Autodesk Inventor part; units mm, degrees
ref_plane "YZ Plane" through (0, 0, 0) normal (1, 0, 0) x (0, 1, 0)
ref_plane "XZ Plane" through (0, 0, 0) normal (0, 1, 0) x (-1, 0, 0)
ref_plane "XY Plane" through (0, 0, 0) normal (0, 0, 1) x (1, 0, 0)
sketch "Sketch1" plane through (0, 0, 0) normal (0, 0, 1) x (1, 0, 0)
  circle A0 centre (0, 0) radius 19
  dimension "d0" = 38
extrude "Extrusion1" add sketch "Sketch1" along normal blind 59.1
sketch "Sketch2" plane through (0, 0, 59.1) normal (0, 0, 1) x (1, 0, 0)
  circle A0 centre (0, 0) radius 16
  dimension "d3" = 32
extrude "Extrusion2" add sketch "Sketch2" along normal blind 41.9
sketch "Sketch3" plane through (0, 0, 101) normal (0, 0, 1) x (1, 0, 0)
  circle A0 centre (0, 0) radius 10
  dimension "d6" = 20
extrude "Extrusion3" add sketch "Sketch3" along normal blind 3
sketch "Sketch4" plane through (0, 0, 104) normal (0, 0, 1) x (1, 0, 0)
  circle A0 centre (0, 0) radius 3
  dimension "d9" = 6
extrude "Extrusion4" add sketch "Sketch4" along normal blind 15.5
sketch "Sketch5" plane through (0, 0, 104) normal (0, 0, 1) x (1, 0, 0)
  line L0 (-9, -9) -> (9, -9) construction
  line L1 (9, -9) -> (9, 9) construction
  line L2 (9, 9) -> (-9, 9) construction
  line L3 (-9, 9) -> (-9, -9) construction
  line L4 (-9, -9) -> (9, 9) construction
  line L5 (9, -9) -> (-9, 9) construction
  circle A0 centre (9, 9) radius 1.5
  circle A1 centre (9, -9) radius 1.5
  circle A2 centre (-9, -9) radius 1.5
  circle A3 centre (-9, 9) radius 1.5
  point P0 (0, 0)
  dimension "d12" = 18
  dimension "d13" = 18
  dimension "d14" = 3
  dimension "d15" = 3
  dimension "d16" = 3
  dimension "d17" = 3
extrude "Extrusion5" cut sketch "Sketch5" against normal blind 25
sketch "Sketch6" plane through (0, 0, 101) normal (0, 0, 1) x (1, 0, 0)
  circle A0 centre (0, 0) radius 3
  circle A1 centre (0, 0) radius 10
  line L0 (-4.3589, -9) -> (4.3589, -9)
  line L1 (-4.3589, 9) -> (4.3589, 9)
  dimension "d20" = 18
extrude "Extrusion6" cut sketch "Sketch6" along normal through all contours L1 A1 | A1 L0
properties part number "12RPM Gear Motor"
Read the model definition and answer for the solid it produces. Units are mm, in the model's axes. A direction names the side the tool comes from. Give positions to 0.01 mm unless a question says otherwise; leave off trailing zeros. Write each loop counter-clockwise with the first axis right and the second up, starting at its lowest first coordinate (ties: lowest second). Pieces come first, ordered by that corner, then holes. Notation, with made-up numbers: (-28.5, -20) - (-0.5, -20) arc R27 ccw to (-0.5, 17) - close; hole circle Ø11 at (-11.5, 89.5). An arc over 180 degrees is marked (long way). Use CSV: the item, a comma, the result in double quotes. Start each with the question number.
(1) Find section C-C (z = 98). Give the vertices of the cut face in (x, y), plus the area to 3 significant figures.
(2) Find section B-B (x = 0). Give the vertices of the cut face in (y, z), plus the area to 3 significant figures.
(3) For faces 1 (the cylindrical face through (-10.2, -9.9, 90.2)), 2 (the cylindrical face through (-10, 0, 102)), 3 (the cylindrical face through (8.767, 16.856, 29.136)), determine the directions among +Z, -Z, +X, -X, +Y, -Y from which every point of the face is accessible in a straight line to the end or side of a thin tool.
(4) Find section D-D (z = 26.5). Give the vertices of the cut face in (x, y).
(5) Find section A-A (y = 0). Give the vertices of the cut face in (x, z).
(6) Given P1, Ø1.5, axis at x = 4, z = 55, coming from the -Y side; P2, Ø10, axis at x = 8, y = 3, coming from the +Z side; P3, Ø12, axis at y = -12.5, z = 19, coming from the +X side, each flat-ended and moving along its own axis, determine where each tip first touches the part or whether it passes through.
(7) Consider line 1 along Y through (x, z) = (-9, 92); line 2 along Z through (x, y) = (2, 8); line 3 along Z through (x, y) = (11.5, 2.5). Determine where each line is inside the solid, lowest interval first.
(8) Determine the mould class of faces 4 (the cylindrical face through (7.8, 8.1, 90.2)), 5 (the flat face through (0, -10, 101)), 6 (the flat face through (0, -9, 102)), 7 (the flat face through (0, 9, 102)) for opening direction Y: +Y half, -Y half, draft (parallel to the pull), parting line (faces both ways), or undercut.
Findings below:
1,outline,"circle Ø32 at (0, 0); hole circle Ø3 at (-9, -9); hole circle Ø3 at (-9, 9); hole circle Ø3 at (9, -9); hole circle Ø3 at (9, 9)"
1,area,"776 mm2"
2,outline,"(-19, 0) - (19, 0) - (19, 59.1) - (16, 59.1) - (16, 101) - (9, 101) - (9, 104) - (3, 104) - (3, 119.5) - (-3, 119.5) - (-3, 104) - (-9, 104) - (-9, 101) - (-16, 101) - (-16, 59.1) - (-19, 59.1) - close"
2,area,"3,730 mm2"
3,face 1,"+Z"
3,face 2,"+Z, -X"
3,face 3,"+Z, -Z"
4,outline,"circle Ø38 at (0, 0)"
5,outline,"(-19, 0) - (19, 0) - (19, 59.1) - (16, 59.1) - (16, 101) - (10, 101) - (10, 104) - (3, 104) - (3, 119.5) - (-3, 119.5) - (-3, 104) - (-10, 104) - (-10, 101) - (-16, 101) - (-16, 59.1) - (-19, 59.1) - close"
6,P1,"y = -18.72"
6,P2,"z = 104"
6,P3,"x = 17.85"
7,line 1,"-13.23 to -10.5, -7.5 to 7.5, 10.5 to 13.23"
7,line 2,"0 to 104"
7,line 3,"0 to 101"
8,face 4,"undercut"
8,face 5,"draft"
8,face 6,"-Y half"
8,face 7,"+Y half"
